from build123d import *

# Parameters (mm, degrees)
SKETCH1_W                    = 190
SKETCH1_H                    = 200
BASE_FLANGE1_DEPTH           = 5
EDGE_FLANGE1_STRIP_W         = 20.4
EDGE_FLANGE1_STRIP_H         = 5
EDGE_FLANGE1_STRIP_CUT_DEPTH = 190
EDGE_FLANGE1_DEPTH           = 190
EDGE_FLANGE2_STRIP_W         = 20.4
EDGE_FLANGE2_STRIP_H         = 5
EDGE_FLANGE2_STRIP_CUT_DEPTH = 190
EDGE_FLANGE2_DEPTH           = 190
CUT_EXTRUDE1_DEPTH           = 171.367250374
CUT_EXTRUDE1_DEPTH_BACK      = 171.367250374
SKETCH12_R                   = 35
CUT_EXTRUDE2_DEPTH           = 171.367250374
CUT_EXTRUDE2_DEPTH_BACK      = 171.367250374
SKETCH13_R                   = 8
CUT_EXTRUDE3_DEPTH           = 243.950612265
CUT_EXTRUDE3_DEPTH_BACK      = 243.950612265
SKETCH14_R                   = 7


# Sheet-metal steps are written as plain solids
with BuildPart() as part:
    # Sketch1 → Base-Flange1 (new body)
    with BuildSketch(Plane.XY):
        Rectangle(SKETCH1_W, SKETCH1_H)
    extrude(amount=-BASE_FLANGE1_DEPTH)

    # Edge-Flange1 strip (across the edge) → Edge-Flange1 strip cut (cut)
    with BuildSketch(Plane(origin=(-95, 100, -5), x_dir=(0, -1, 0), z_dir=(1, 0, 0))):
        with Locations((-5, -2.5)):
            Rectangle(EDGE_FLANGE1_STRIP_W, EDGE_FLANGE1_STRIP_H)
    extrude(amount=EDGE_FLANGE1_STRIP_CUT_DEPTH, mode=Mode.SUBTRACT)

    # Edge-Flange1 section (across the edge) → Edge-Flange1 (add)
    with BuildSketch(Plane(origin=(-95, 100, -5), x_dir=(0, -1, 0), z_dir=(1, 0, 0))):
        with BuildLine():
            Line((0, 0.2), (0, 95))
            Line((0, 95), (5, 95))
            Line((5, 95), (5, 0.2))
            ThreePointArc((5, 0.2), (5.058578644, 0.058578644), (5.2, 0))
            Line((5.2, 0), (5.2, -5))
            ThreePointArc((5.2, -5), (1.523044738, -3.476955262), (0, 0.2))
        make_face()
    extrude(amount=EDGE_FLANGE1_DEPTH)

    # Edge-Flange2 strip (across the edge) → Edge-Flange2 strip cut (cut)
    with BuildSketch(Plane(origin=(95, -100, -5), x_dir=(0, 1, 0), z_dir=(-1, 0, 0))):
        with Locations((-5, -2.5)):
            Rectangle(EDGE_FLANGE2_STRIP_W, EDGE_FLANGE2_STRIP_H)
    extrude(amount=EDGE_FLANGE2_STRIP_CUT_DEPTH, mode=Mode.SUBTRACT)

    # Edge-Flange2 section (across the edge) → Edge-Flange2 (add)
    with BuildSketch(Plane(origin=(95, -100, -5), x_dir=(0, 1, 0), z_dir=(-1, 0, 0))):
        with BuildLine():
            Line((0, 0.2), (0, 95))
            Line((0, 95), (5, 95))
            Line((5, 95), (5, 0.2))
            ThreePointArc((5, 0.2), (5.058578644, 0.058578644), (5.2, 0))
            Line((5.2, 0), (5.2, -5))
            ThreePointArc((5.2, -5), (1.523044738, -3.476955262), (0, 0.2))
        make_face()
    extrude(amount=EDGE_FLANGE2_DEPTH)

    # Sketch12 → Cut-Extrude1 (cut, two sides: drawn at the far end of the back side and taken through both)
    with BuildSketch(Plane.XY.offset(-CUT_EXTRUDE1_DEPTH_BACK)):
        with Locations(Location((0, 0, 0), (0, 0, 180))):
            Circle(SKETCH12_R)
    extrude(amount=CUT_EXTRUDE1_DEPTH + CUT_EXTRUDE1_DEPTH_BACK, mode=Mode.SUBTRACT)

    # Sketch13 → Cut-Extrude2 (cut, two sides: drawn at the far end of the back side and taken through both)
    with BuildSketch(Plane.XY.offset(-CUT_EXTRUDE2_DEPTH_BACK)):
        with Locations(Location((55.5, 55.5, 0), (0, 0, 180))):
            Circle(SKETCH13_R)
        with Locations(Location((-55.5, 55.5, 0), (0, 0, 180))):
            Circle(SKETCH13_R)
        with Locations(Location((-55.5, -55.5, 0), (0, 0, 180))):
            Circle(SKETCH13_R)
        with Locations(Location((55.5, -55.5, 0), (0, 0, 180))):
            Circle(SKETCH13_R)
    extrude(amount=CUT_EXTRUDE2_DEPTH + CUT_EXTRUDE2_DEPTH_BACK, mode=Mode.SUBTRACT)

    # Sketch14 → Cut-Extrude3 (cut, two sides: drawn at the far end of the back side and taken through both)
    with BuildSketch(Plane(origin=(0, -100, 0), x_dir=(-1, 0, 0), z_dir=(0, -1, 0)).offset(-CUT_EXTRUDE3_DEPTH_BACK)):
        with Locations(Location((75, 85, 0), (0, 0, 270))):
            Circle(SKETCH14_R)
        with Locations(Location((-75, 85, 0), (0, 0, 270))):
            Circle(SKETCH14_R)
    extrude(amount=CUT_EXTRUDE3_DEPTH + CUT_EXTRUDE3_DEPTH_BACK, mode=Mode.SUBTRACT)


solid = part.part
Part model, mm, in its own coordinate system. A direction names the side the tool comes from. Give positions to 0.01 mm unless a question says otherwise; leave off trailing zeros. Write each loop counter-clockwise with the first axis right and the second up, starting at its lowest first coordinate (ties: lowest second). Pieces come first, ordered by that corner, then holes.
1) Cut at B-B on y = 0. Write the cut outline in (x, z).
Resolved:
outline: (-95, -5) - (-35, -5) - (-35, 0) - (-95, 0) - close; (35, -5) - (95, -5) - (95, 0) - (35, 0) - close
2) Two-plate mould, pull along Z, no slides. Class faces 1 (the face through (70.27, -97.46, -90.16)), 2 (the face through (-95, 0, -2)), 3 (the face through (-1, 98, -100)): released by +Z, released by -Z, zero draft, split by the parting line, or undercut.
Resolved:
face 1: undercut
face 2: zero draft
face 3: released by -Z
3) Pin check, flat tips, straight feed: pin 1 (12.5 mm diameter, centred on x = -75, z = -85, fed in from +Y); pin 2 (12 mm diameter, centred on x = 72.5, y = -6.5, fed in from -Z). Stop position of each tip, or through.
Resolved:
pin 1: passes through
pin 2: stops at z = -5
4) Cut at A-A on x = 75. Write the cut outline in (y, z).
Resolved:
outline: (-100, -100) - (-95, -100) - (-95, -92) - (-100, -92) - close; (-100, -78) - (-95, -78) - (-95, -5.2) arc R0.2 cw to (-94.8, -5) - (94.8, -5) arc R0.2 cw to (95, -5.2) - (95, -78) - (100, -78) - (100, -5.2) arc R5.2 ccw to (94.8, 0) - (-94.8, 0) arc R5.2 ccw to (-100, -5.2) - close; (95, -100) - (100, -100) - (100, -92) - (95, -92) - close
5) Probe L1, parallel to X at y = -96.6, z = -85; L2, parallel to Y at x = -15, z = -47; L3, parallel to Y at x = 55.5, z = -1.3. List the from-to ranges inside material, lowest first.
Resolved:
L1: x = -95 to -82, -68 to 68, 82 to 95
L2: y = -100 to -95, 95 to 100
L3: y = -98.24 to -63.5, -47.5 to 47.5, 63.5 to 98.24
6) Cut at D-D on x = 0. Write the cut outline in (y, z).
Resolved:
outline: (-100, -100) - (-95, -100) - (-95, -5.2) arc R0.2 cw to (-94.8, -5) - (-35, -5) - (-35, 0) - (-94.8, 0) arc R5.2 ccw to (-100, -5.2) - close; (35, -5) - (94.8, -5) arc R0.2 cw to (95, -5.2) - (95, -100) - (100, -100) - (100, -5.2) arc R5.2 ccw to (94.8, 0) - (35, 0) - close
7) Cut at C-C on z = -16.5. Write the cut outline in (x, y), then the cut area to 3 significant figures.
Resolved:
outline: (-95, -100) - (95, -100) - (95, -95) - (-95, -95) - close; (-95, 95) - (95, 95) - (95, 100) - (-95, 100) - close
area: 1,900 mm2
8) Which spindle directions (+Z, -Z, +X, -X, +Y, -Y) get a long thin tool onto all of the face, cutting with end or side? Do faces 4 (the face through (1, -100, -52)), 5 (the face through (-1, 95, -53)). Say none if no direction does.
Resolved:
face 4: +Z, -Z, +X, -X, -Y
face 5: -Z, +X, -X
